Verification items for the finished model (mm, model axes). Face numbers are marked on the shaded views. A direction names the side the tool comes from. Round coordinates to 2 decimals unless told otherwise and drop trailing zeros. Order: outer loops, then holes, each group sorted by start corner. A loop starts at its lowest first (then second) coordinate and runs counter-clockwise, first axis right, second up.
```python
from build123d import *

# Parameters (mm, degrees)
F1_DEPTH = 39.5


with BuildPart() as f1:
    # F0 (on Front) → F1 (new body)
    with BuildSketch(Plane.XZ):
        Polygon((0, 75), (0, 0), (3.6, 0), (10.06858, 0), (4.592586, 75), align=None)
        Polygon((3.6, 0), (0, 0), (0, -53), (3.6, -53), (3.6, -50), (3.6, -42.764902), (3.6, -5.754051), align=None)
        Polygon((10.06858, 0), (3.6, 0), (3.6, -5.754051), (26.496561, 0), align=None)
        Polygon((15.96995, -50), (3.6, -42.764902), (3.6, -50), align=None)
    extrude(amount=F1_DEPTH)


solid = f1.part
```
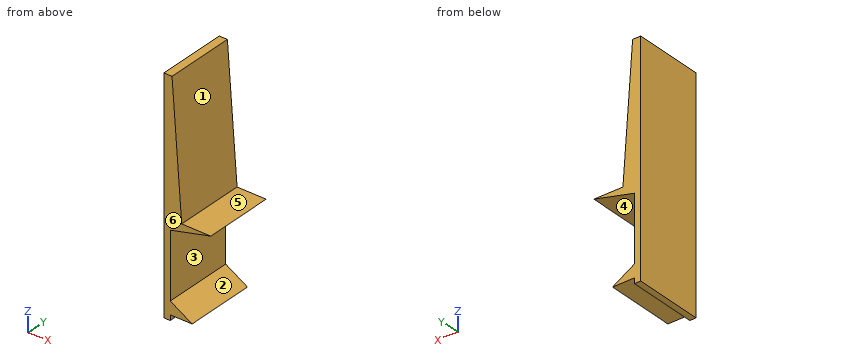
1) Sectioned sample at D-D on x = 21.25. Record the cut outline in (y, z).
2) Sectioned sample at C-C on z = -25. Record the cut outline in (x, y).
3) Scan lines: probe 1 along X at (y, z) = (-9, -11); probe 2 along Z at (x, y) = (4, -29); probe 3 along X at (y, z) = (-27, 32.5). Record each from-to range of solid material in increasing order.
4) Sectioned sample at B-B on y = -3.5. Record the cut outline in (x, z).
5) Sectioned sample at A-A on x = 13. Record the cut outline in (y, z), then the cut area to 3 significant figures.
6) Tool access check on the marked faces 1 and 2. Record the directions out of +Z, -Z, +X, -X, +Y, -Y that give a thin tool (end or side, any length) a straight path to the whole face; none if there is none.
7) Draft check along Z on the marked faces 3, 4, 5 and 6. Enter one of: released by +Z, released by -Z, zero draft, split by the parting line, or undercut.
8) Go/stop test with flat-tipped pins: pin 1 Ø10 at (y, z) = (-14, 47.5) entering from -X; pin 2 Ø8 at (y, z) = (-33.5, 20) entering from +X; pin 3 Ø2 at (x, y) = (22, -16) entering from +Z; pin 4 Ø6 at (x, y) = (7.5, -12.5) entering from -Z. Record where each tip stops, or that it passes through.
Returned:
1. outline: (-39.5, -1.32) - (0, -1.32) - (0, 0) - (-39.5, 0) - close
2. outline: (0, -39.5) - (3.6, -39.5) - (3.6, 0) - (0, 0) - close
3. probe 1: x = 0 to 3.6
3. probe 2: z = -50 to -43, -5.65 to 75
3. probe 3: x = 0 to 7.7
4. outline: (0, -53) - (3.6, -53) - (3.6, -50) - (15.97, -50) - (3.6, -42.76) - (3.6, -5.75) - (26.5, 0) - (10.07, 0) - (4.59, 75) - (0, 75) - close
5. outline: (-39.5, -50) - (0, -50) - (0, -48.26) - (-39.5, -48.26) - close; (-39.5, -3.39) - (0, -3.39) - (0, 0) - (-39.5, 0) - close
5. area: 203 mm2
6. face 1: +Z, +X, +Y, -Y
6. face 2: +X, +Y, -Y
7. face 3: undercut
7. face 4: undercut
7. face 5: released by +Z
7. face 6: zero draft
8. pin 1: stops at x = 0
8. pin 2: stops at x = 8.9
8. pin 3: stops at z = 0
8. pin 4: stops at z = -50
